```python
from build123d import *

# Parameters (mm, degrees)
F1_DEPTH = 30
F2_W     = 10
F2_H     = 10
F3_DEPTH = 8
F4_R     = 4.99999


# Not quite as in the source:
# - a fillet or chamfer is up to 0.001 mm smaller than in the source, because OpenCascade refuses the exact size


with BuildPart() as f1:
    # F0 (on Front) → F1 (new body)
    with BuildSketch(Plane.XZ):
        with BuildLine():
            ThreePointArc((-15, 0), (0, 15), (15, 0))
            Line((15, 0), (45, 0))
            Line((45, 0), (45, 25))
            Line((45, 25), (37, 25))
            Line((37, 25), (37, 8))
            Line((37, 8), (21.5638586528, 8))
            ThreePointArc((21.5638586528, 8), (-4.0639421123, 22.6381177333), (-23, 0))
            Line((-23, 0), (-15, 0))
        make_face()
    extrude(amount=F1_DEPTH)

    # F2 (on face) → F3 (cut, through all)
    with BuildSketch(Plane.YZ.offset(45)):
        with Locations((-15, 20)):
            Rectangle(F2_W, F2_H)
    extrude(amount=-F3_DEPTH, mode=Mode.SUBTRACT)

    # F4 (radius 5 in the source; OpenCascade refuses exactly that, so slightly less here)
    f4_edges = [f1.edges().sort_by_distance(p)[0] for p in [
        (41, -30, 25),
        (41, 0, 25),
        (41, -10, 15),
        (41, -20, 15),
    ]]
    fillet(f4_edges, radius=F4_R)


solid = f1.part
```
Input: part model. Units: mm. Frame: model coordinates. A direction names the side the tool comes from. Coordinates: 2 decimals unless noted, no trailing zeros. Loops run counter-clockwise (first coordinate to the right, second up) from the corner with the lowest first, then second, coordinate; pieces in that order, holes last. Notation, with made-up numbers: M -10,22.25 L 40,22.25 A13 ccw 40,31.25 Z; hole C -22,55.25 d5. An arc over 180 degrees is marked long. Use a Markdown table: item, result. Add a question column.
1) Line query: L1, parallel to X at y = -23, z = 12.5; L2, parallel to X at y = -14, z = 10.5; L3, parallel to X at y = -5.25, z = 2. Output: solid intervals per line, ascending. Write a range as from..to.
2) Set-up query: faces 5 (the flat face through (37, -14.8, 14.7)), 6 (the cylindrical face through (41, -29, 23)), 7 (the cylindrical face through (41, -11, 17)), 8 (the flat face through (30, -15, 0)). Return all of +Z, -Z, +X, -X, +Y, -Y with unobstructed straight access to the full face (end or side cutting, diameter ignored); none if empty.
3) Draft query along Y for faces 1 (the cylindrical face through (41, -18, 16)), 2 (the flat face through (41, -20, 22)), 3 (the cylindrical face through (41, -1, 23)), 4 (the flat face through (41, -7, 25)). Return one class per face: +Y half, -Y half, draft (parallel to the pull), parting line (faces both ways), or undercut.
4) Section D-D, the plane z = 21.75. Return the cut outline in (x, y), plus the area to 3 significant figures.
5) Section A-A, the plane z = 17.5. Return the cut outline in (x, y).
6) Section C-C, the plane y = -21. Return the cut outline in (x, z).
7) Pin query (flat end, axial travel): P1, Ø1, axis at y = -16.5, z = 20, coming from the -X side; P2, Ø10, axis at y = -19, z = 6, coming from the -X side; P3, Ø5.5, axis at x = 42, z = 23.5, coming from the +Y side. Return the tip coordinate at first contact, or that it passes through.
Answer below:
| question | item | result |
|---|---|---|
| 1 | L1 | -19.31..-8.29, 8.29..19.31, 37..45 |
| 1 | L2 | -20.46..-10.71, 10.71..20.46, 37..45 |
| 1 | L3 | -22.91..-14.87, 14.87..45 |
| 2 | face 5 | +Z, +Y, -Y |
| 2 | face 6 | +Z, +X, -Y |
| 2 | face 7 | +Z, +X |
| 2 | face 8 | -Z, +X, -X, +Y, -Y |
| 3 | face 1 | undercut |
| 3 | face 2 | undercut |
| 3 | face 3 | +Y half |
| 3 | face 4 | draft |
| 4 | outline | M -7.48,-30 L 7.48,-30 L 7.48,0 L -7.48,0 Z; M 37,-29.68 L 45,-29.68 L 45,-20 L 37,-20 Z; M 37,-10 L 45,-10 L 45,-0.32 L 37,-0.32 Z |
| 4 | area | 604 mm2 |
| 5 | outline | M -14.92,-30 L 14.92,-30 L 14.92,0 L -14.92,0 Z; M 37,-30 L 45,-30 L 45,-19.33 L 37,-19.33 Z; M 37,-10.67 L 45,-10.67 L 45,0 L 37,0 Z |
| 6 | outline | M -23,0 L -15,0 A15 cw 15,0 L 45,0 L 45,25 L 37,25 L 37,8 L 21.56,8 A23 ccw Z |
| 7 | P1 | x = -12.2 |
| 7 | P2 | x = -22.98 |
| 7 | P3 | y = -0.06 |
